Could you check a few things on this model? Use its own coordinates, in mm. Round coordinates to 2 decimals unless told otherwise and drop trailing zeros. Answer in a Markdown table with one row per item.
from build123d import *

# Parameters (mm, degrees)
F0_R      = 2.5
F1_DEPTH  = 0.5
F2_R      = 1
F2_R_2    = 0.7
F3_DEPTH  = 14
F5_DEPTH  = 0.5
F6_R      = 0.15
F7_R      = 3
F7_R_2    = 2.5
F10_DEPTH = 100
F11_R     = 0.6
F12_DEPTH = 2


with BuildPart() as f1:
    # F0 (on Front) → F1 (new body)
    with BuildSketch(Plane.XZ):
        Circle(F0_R)
    extrude(amount=F1_DEPTH)

    # F2 (on face) → F3 (join)
    with BuildSketch(Plane(origin=(0, 0, 0), x_dir=(-1, 0, 0), z_dir=(0, 1, 0))):
        Circle(F2_R)
        Circle(F2_R_2, mode=Mode.SUBTRACT)
    extrude(amount=F3_DEPTH)

    # F4 (on face) → F5 (join)
    with BuildSketch(Plane(origin=(0, 14, 0), x_dir=(-1, 0, 0), z_dir=(0, 1, 0))):
        with BuildLine():
            ThreePointArc((-2.49769, 0.107441), (-2.075, 0), (-2.49769, -0.107441))
            ThreePointArc((-2.49769, -0.107441), (2.5, 0), (-2.49769, 0.107441))
        make_face()
    extrude(amount=F5_DEPTH)

    # F9: sweep along a path in F8
    with BuildLine(Plane.XY) as f9_path:
        Line((2.35, 0), (2.286365, 14.495411))
        ThreePointArc((2.286365, 14.495411), (2.286324, 14.5), (2.286241, 14.504588))
        Line((2.286241, 14.504588), (0.000129, 114.994315))
        ThreePointArc((0.000129, 114.994315), (3.2e-05, 115), (0, 115.005687))
        Line((0, 115.005687), (0, 121.5))
    # F6 (on face) → F9 (sweep)
    with BuildSketch(Plane(origin=(0, 0, 0), x_dir=(-1, 0, 0), z_dir=(0, 1, 0))):
        with Locations((-2.35, 0)):
            Circle(F6_R)
    sweep(path=f9_path.line)

    # F7 (on face) → F10 (join)
    with BuildSketch(Plane.XZ.offset(-14)):
        Circle(F7_R)
        Circle(F7_R_2, mode=Mode.SUBTRACT)
    extrude(amount=-F10_DEPTH)

    # F11 (on face) → F12 (join)
    with BuildSketch(Plane(origin=(0.533374, 121.497658, 0), x_dir=(-0.99999, 0.00439, 0), z_dir=(0.00439, 0.99999, 0))):
        with BuildLine():
            Line((5.217127, 1.75), (-4.15037, 1.75))
            ThreePointArc((-4.15037, 1.75), (-4.466621, 0), (-4.15037, -1.75))
            Line((-4.15037, -1.75), (5.217127, -1.75))
            ThreePointArc((5.217127, -1.75), (5.533379, 0), (5.217127, 1.75))
        make_face()
        with Locations((-2.466621, 0)):
            Circle(F11_R, mode=Mode.SUBTRACT)
        with Locations((3.533379, 0)):
            Circle(F11_R, mode=Mode.SUBTRACT)
    extrude(amount=-F12_DEPTH)


solid = f1.part
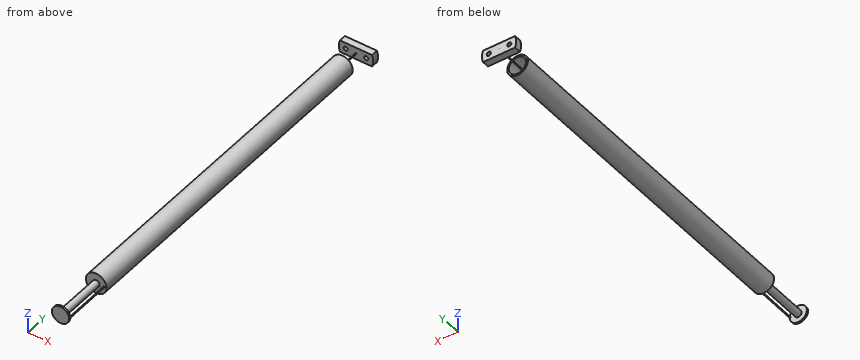
1) Please list where these lines run through material, in increasing order: line 1 (Y direction, x = -1.5, z = -1.4); line 2 (Z direction, x = 0, y = 53); line 3 (Z direction, x = 0, y = 7.5).
Findings:
| item | result |
|---|---|
| line 1 | y = -0.5 to 0, 14 to 14.5, 119.51 to 121.51 |
| line 2 | z = -3 to -2.5, 2.5 to 3 |
| line 3 | z = -1 to -0.7, 0.7 to 1 |
2) For pin 1 (1.5 mm diameter, centred on x = 0, z = 0, fed in from +Y); pin 2 (1.5 mm diameter, centred on y = 19, z = -0.5, fed in from +X); pin 3 (2 mm diameter, centred on x = -2, y = 120, fed in from -Z), each with a flat end and sliding along its axis, tell me the tip position at first contact or that it passes through.
Findings:
| item | result |
|---|---|
| pin 1 | stops at y = 121.5 |
| pin 2 | stops at x = 3 |
| pin 3 | stops at z = -1.75 |
3) Imagine slicing it at A-A, the plane y = 25.5. Count the separate pieces of the cut face and the enclosed holes in it, plus the area to 3 significant figures.
Findings:
| item | result |
|---|---|
| separate pieces | 2 |
| enclosed holes | 1 |
| area | 8.71 mm^2 |
